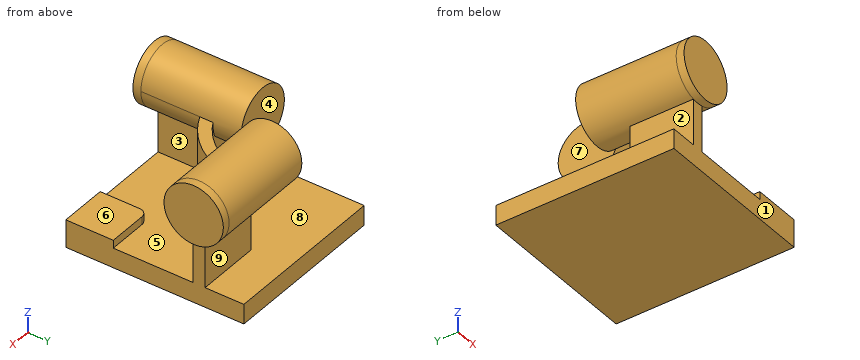
from build123d import *

# Parameters (mm, degrees)
F0_W          = 210
F0_H          = 225
F1_DEPTH      = 25
F3_DEPTH      = 95
F4_R          = 37.5
F5_DEPTH      = 10
F5_DEPTH_BACK = 127
F6_R          = 37.5
F7_DEPTH      = 10
F7_DEPTH_BACK = 127
F8_W          = 60
F8_H          = 60
F9_DEPTH      = 10
F10_R         = 10


with BuildPart() as f1:
    # F0 (on Top) → F1 (new body)
    with BuildSketch(Plane.XY):
        Rectangle(F0_W, F0_H)
    extrude(amount=F1_DEPTH)

    # F2 (on face) → F3 (join)
    with BuildSketch(Plane.XY.offset(25)):
        with BuildLine():
            Line((-71, -32.5), (-71, -112.5))
            Line((-71, -112.5), (-56, -112.5))
            Line((-56, -112.5), (-56, -46.481817))
            ThreePointArc((-56, -46.481817), (7.488853, -14.988853), (38.981817, 48.5))
            Line((38.981817, 48.5), (105, 48.5))
            Line((105, 48.5), (105, 63.5))
            Line((105, 63.5), (25, 63.5))
            ThreePointArc((25, 63.5), (-3.117749, -4.382251), (-71, -32.5))
        make_face()
    extrude(amount=F3_DEPTH)

    # F4 (on face) → F5 (join, two sides)
    with BuildSketch(Plane.XZ.offset(112.5)) as f5_sk:
        with Locations((-63.5, 120)):
            Circle(F4_R)
    extrude(amount=F5_DEPTH)
    extrude(f5_sk.sketch, amount=-F5_DEPTH_BACK)

    # F6 (on face) → F7 (join, two sides)
    with BuildSketch(Plane.YZ.offset(105)) as f7_sk:
        with Locations((56.305401, 120.402195)):
            Circle(F6_R)
    extrude(amount=F7_DEPTH)
    extrude(f7_sk.sketch, amount=-F7_DEPTH_BACK)

    # F8 (on face) → F9 (join)
    with BuildSketch(Plane.XY.offset(25)):
        with Locations((75, -82.5)):
            Rectangle(F8_W, F8_H)
    extrude(amount=F9_DEPTH)

    # F10
    f10_edges = [f1.edges().sort_by_distance(p)[0] for p in [
        (45, -52.5, 30),
    ]]
    fillet(f10_edges, radius=F10_R)


solid = f1.part
Input: part model. Units: mm. Frame: model coordinates. Face numbers are marked on the shaded views. A direction names the side the tool comes from. Give positions to 0.01 mm unless a question says otherwise; leave off trailing zeros. Order: outer loops, then holes, each group sorted by start corner. A loop starts at its lowest first (then second) coordinate and runs counter-clockwise, first axis right, second up. Notation, with made-up numbers: (65.25, -30) - (91.25, -30) arc R24 cw to (91.25, -10) - close; hole circle Ø2 at (39, 89.5). An arc over 180 degrees is marked (long way). Answer as a JSON object with one key per item and string values. Group by question number.
Q1. Line query: probe 1 along X at (y, z) = (-92.5, 26); probe 2 along Y at (x, z) = (28.5, 7); probe 3 along Z at (x, y) = (57, 35). Output: solid intervals per line, ascending.
Q2. Cut plane D-D, the plane y = 33.5. Output: boundary loops of the cut face in (x, z), then the cut area to 3 significant figures.
Q3. Cut plane B-B, the plane y = -1. Output: boundary loops of the cut face in (x, z), then the cut area to 3 significant figures.
Q4. Cut plane C-C, the plane z = 60.5. Output: boundary loops of the cut face in (x, y).
Q5. First-contact query: pin 1 Ø12 at (x, y) = (-69.5, 84) entering from -Z; pin 2 Ø3 at (x, z) = (9.5, 76.5) entering from +Y; pin 3 Ø4 at (y, z) = (47, 79.5) entering from -X; pin 4 Ø4 at (y, z) = (53, 58) entering from +X. Flat tips, straight axial feed; report the tip coordinate or a pass-through.
Q6. Cut plane A-A, the plane x = -86.5. Output: boundary loops of the cut face in (y, z), then the cut area to 3 significant figures.
Q7. Mould query, pull axis Z, two halves, no side actions, for the marked faces 6, 7, 8 and 9. Classes: pulls with the +Z half, pulls with the -Z half, needs draft (parallel to the pull), parting line crosses it, or undercut.
Q8. Set-up query: the marked faces 1, 2, 3, 4 and 5. Return all of +Z, -Z, +X, -X, +Y, -Y with unobstructed straight access to the full face (end or side cutting, diameter ignored); none if empty.
Results:
{
 "1": {"probe 1": "-71 to -56, 45 to 105", "probe 2": "-112.5 to 112.5", "probe 3": "0 to 25, 89.54 to 151.26"},
 "2": {"outline": "(-105, 0) - (105, 0) - (105, 25) - (35.87, 25) - (35.87, 90.63) - (115, 90.63) - (115, 150.17) - (-22, 150.17) - (-22, 90.63) - (20.19, 90.63) - (20.19, 25) - (-105, 25) - close", "area": "14,400 mm^2"},
 "3": {"outline": "(-105, 0) - (105, 0) - (105, 25) - (19.34, 25) - (19.34, 120) - (0.1, 120) - (0.1, 25) - (-105, 25) - close; circle Ø75 at (-63.5, 120)", "area": "11,500 mm^2"},
 "4": {"outline": "(-71, -112.5) - (-56, -112.5) - (-56, -46.48) arc R111 ccw to (38.98, 48.5) - (105, 48.5) - (105, 63.5) - (25, 63.5) arc R96 cw to (-71, -32.5) - close"},
 "5": {"pin 1": "z = 0", "pin 2": "y = 13.58", "pin 3": "x = 23.2", "pin 4": "x = 105"},
 "6": {"outline": "(-122.5, 90.38) - (14.5, 90.38) - (14.5, 149.62) - (-122.5, 149.62) - close; (-112.5, 0) - (112.5, 0) - (112.5, 25) - (-112.5, 25) - close", "area": "13,700 mm^2"},
 "7": {"face 6": "pulls with the +Z half", "face 7": "needs draft", "face 8": "undercut", "face 9": "undercut"},
 "8": {"face 1": "-Z, +X, -X, -Y", "face 2": "-X, +Y, -Y", "face 3": "-Y", "face 4": "+Z, -X, +Y", "face 5": "none"}
}
